Geometry check sheet. Reference: drawing and pictorial views, mm from the part's lowest x, y, z. A direction names the side the tool comes from. Coordinates: 2 decimals unless noted, no trailing zeros. Loops run counter-clockwise (first coordinate to the right, second up) from the corner with the lowest first, then second, coordinate; pieces in that order, holes last. Notation, with made-up numbers: (76.5, 41.5) -> (129.5, 41.5) arc R25 ccw to (129.5, 60.5) -> close; hole circle Ø8 at (-18.5, 52). An arc over 180 degrees is marked (long way). Answer as a JSON object with one key per item and string values. Group by question number.
Q1. Cross-section at A-A on y = 10.5. Record the boundary of the cut face in (x, z), and give its area (3 significant figures).
Q2. Set-up check for the marked faces 1, 2, 3 and 4: record each of +Z, -Z, +X, -X, +Y, -Y from which the full face is reachable in a straight line by a thin tool's end or side.
Q3. Scan lines: L1, parallel to X at y = 6.75, z = 7; L2, parallel to Z at x = 51, y = 18. Record each from-to range of solid material in increasing order.
Q4. Cross-section at B-B on x = 5. Record the boundary of the cut face in (y, z), and give its area (3 significant figures).
Q5. Gauge pin test, flat ends, axial feed: pin 1 Ø9.5 at (x, y) = (11, 5.5) entering from +Z; pin 2 Ø1.5 at (x, z) = (30.5, 11.5) entering from -Y; pin 3 Ø4 at (y, z) = (15.5, 17) entering from +X; pin 4 Ø5 at (y, z) = (10, 50.5) entering from -X. Record the tip position at first contact, or that the pin passes through.
Q6. Cross-section at C-C on z = 49.5. Record the boundary of the cut face in (x, y), and give its area (3 significant figures).
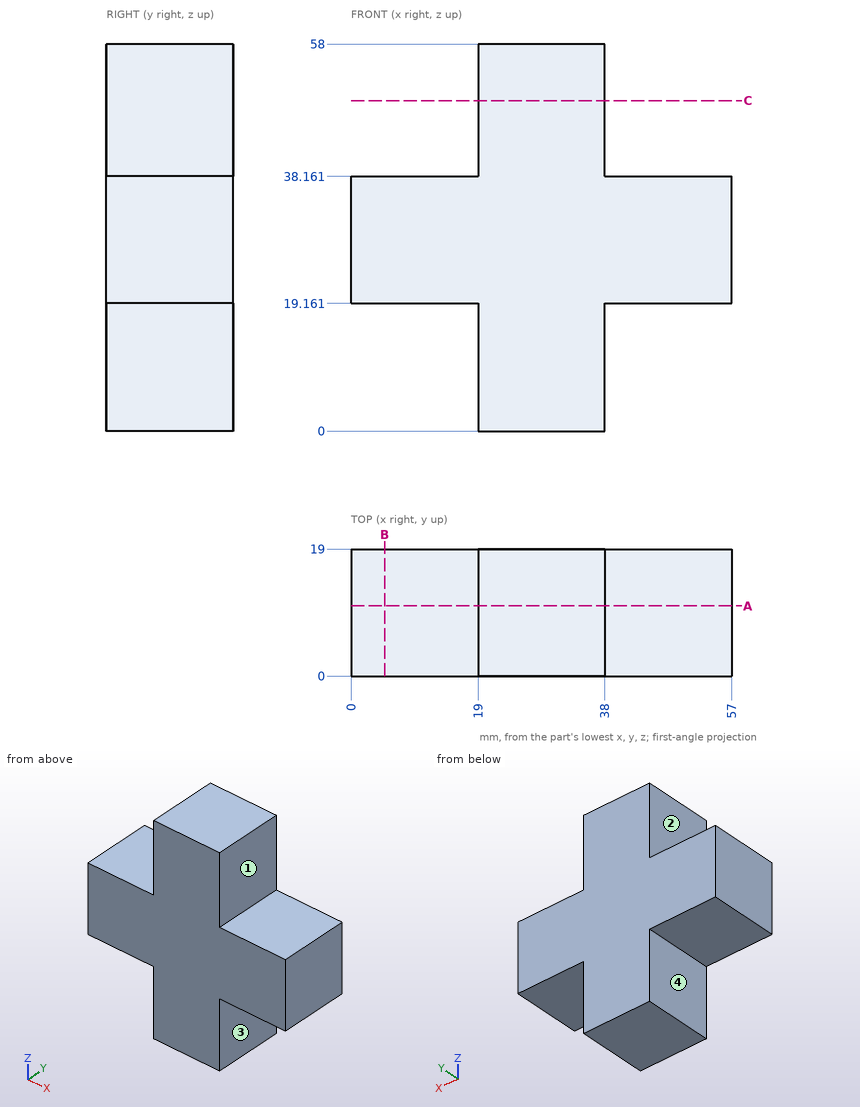
Computed values:
{
 "1": {"outline": "(0, 19.16) -> (19, 19.16) -> (19, 0) -> (38, 0) -> (38, 19.16) -> (57, 19.16) -> (57, 38.16) -> (38, 38.16) -> (38, 58) -> (19, 58) -> (19, 38.16) -> (0, 38.16) -> close", "area": "1,820 mm²"},
 "2": {"face 1": "+Z, +X, +Y, -Y", "face 2": "+Z, -X, +Y, -Y", "face 3": "-Z, +X, +Y, -Y", "face 4": "-Z, -X, +Y, -Y"},
 "3": {"L1": "x = 19 to 38", "L2": "z = 19.16 to 38.16"},
 "4": {"outline": "(0, 19.16) -> (19, 19.16) -> (19, 38.16) -> (0, 38.16) -> close", "area": "361 mm²"},
 "5": {"pin 1": "stops at z = 38.16", "pin 2": "stops at y = 0", "pin 3": "stops at x = 38", "pin 4": "stops at x = 19"},
 "6": {"outline": "(19, 0) -> (38, 0) -> (38, 19) -> (19, 19) -> close", "area": "361 mm²"}
}
